Could you check a few things on this model? Use its own coordinates, in mm. A direction names the side the tool comes from. Round coordinates to 2 decimals unless told otherwise and drop trailing zeros. Write each loop counter-clockwise with the first axis right and the second up, starting at its lowest first coordinate (ties: lowest second). Pieces come first, ordered by that corner, then holes. Notation, with made-up numbers: (83.5, 50) -> (97.5, 50) arc R23 cw to (97.5, 61) -> close; hole circle Ø9 at (-34, -27). An arc over 180 degrees is marked (long way). One line per question, with ' | ' between items. Start each with the question number.
1. Imagine slicing it at B-B, the plane x = -85.5. List the corners of the cut face in (y, z) for me, and give its area (3 significant figures).
2. If I drill on line 1 along X through (y, z) = (0.75, -100); line 2 along X through (y, z) = (1.75, 70); line 3 along Z through (x, y) = (0, 1.8), over which ranges is the centre line in solid material (lowest first)? Write a range as [from, to].
3. For faces 1 (the flat face through (-95, 3, -95)), 2 (the flat face through (-53, 3, 123)), 3 (the flat face through (95, 3, -95)), 4 (the flat face through (85, 3, -105)), which set-ups out of +Z, -Z, +X, -X, +Y, -Y let a thin tool reach every point of the face, with its end or its side?
4. Thinking about a two-plate mould opening in X: for faces 5 (the flat face through (-90, 3, 120)), 6 (the flat face through (0, 3, -15)), 7 (the flat face through (-24, 0, -2)), which applies, released by +X, released by -X, zero draft, split by the parting line, or undercut?
5. Imagine slicing it at C-C, the plane y = 1.1. State how many separate pieces and enclosed holes the cut face has, and give its area (3 significant figures).
6. For pin 1 Ø2 at (x, y) = (-47, 1.5) entering from -Z; pin 2 Ø2.5 at (x, z) = (-20.61, 59.52) entering from -Y (1 decimal); pin 3 Ø2 at (x, y) = (-50, 4) entering from -Z, each with a flat end and sliding along its axis, tell me the tip position at first contact or that it passes through.
7. Imagine slicing it at A-A, the plane x = 5. List the corners of the cut face in (y, z) for me, and give its area (4 significant figures).
from build123d import *

# Parameters (mm, degrees)
SKETCH_1_W           = 200
SKETCH_1_H           = 250
EXTRUDE_1_DEPTH      = 5
CUT_EXTRUDE_1_DEPTH  = 35
CUT_EXTRUDE_2_DEPTH  = 35
CUT_EXTRUDE_3_DEPTH  = 35
CUT_EXTRUDE_5_DEPTH  = 30
CUT_EXTRUDE_6_DEPTH  = 10
CUT_EXTRUDE_7_DEPTH  = 10
SKETCH_9_R           = 1.5
CUT_EXTRUDE_8_DEPTH  = 10
SKETCH_10_R          = 1.5
CUT_EXTRUDE_9_DEPTH  = 10
SKETCH_12_R          = 1.5
CUT_EXTRUDE_10_DEPTH = 10
SKETCH_13_R          = 1.5
CUT_EXTRUDE_11_DEPTH = 10


with BuildPart() as part:
    # 草图1 → 凸台-拉伸1 (new body)
    with BuildSketch(Plane(origin=(0, 0, 0), x_dir=(1, 0, 0), z_dir=(0, 1, 0))):
        Rectangle(SKETCH_1_W, SKETCH_1_H)
    extrude(amount=EXTRUDE_1_DEPTH)

    # 草图2 → 切除-拉伸1 (cut)
    with BuildSketch(Plane(origin=(0, 5, 0), x_dir=(1, 0, 0), z_dir=(0, 1, 0))):
        Polygon((-100, -115), (-80, -125), (-100, -125), align=None)
    cut_extrude_1 = extrude(amount=-CUT_EXTRUDE_1_DEPTH, mode=Mode.SUBTRACT)

    # 镜向1: 切除-拉伸1 across plane
    add(cut_extrude_1.mirror(Plane(origin=(0, 0, 0), x_dir=(0, 0, 1), z_dir=(1, 0, 0))), mode=Mode.SUBTRACT)

    # 草图3 → 切除-拉伸2 (cut)
    with BuildSketch(Plane(origin=(0, 5, 0), x_dir=(1, 0, 0), z_dir=(0, 1, 0))):
        Polygon((-55, -125), (-50, -120), (0, -120), (0, -125), align=None)
    cut_extrude_2 = extrude(amount=-CUT_EXTRUDE_2_DEPTH, mode=Mode.SUBTRACT)

    # 镜向2: 切除-拉伸2 across plane
    add(cut_extrude_2.mirror(Plane(origin=(0, 0, 0), x_dir=(0, 0, 1), z_dir=(1, 0, 0))), mode=Mode.SUBTRACT)

    # 草图4 → 切除-拉伸3 (cut)
    with BuildSketch(Plane(origin=(0, 5, 0), x_dir=(1, 0, 0), z_dir=(0, 1, 0))):
        with BuildLine():
            Line((-12.5, -95), (12.5, -95))
            ThreePointArc((12.5, -95), (14.267766953, -95.732233047), (15, -97.5))
            Line((15, -97.5), (15, -107.5))
            ThreePointArc((15, -107.5), (14.267766953, -109.267766953), (12.5, -110))
            Line((12.5, -110), (-12.5, -110))
            ThreePointArc((-12.5, -110), (-14.267766953, -109.267766953), (-15, -107.5))
            Line((-15, -107.5), (-15, -97.5))
            ThreePointArc((-15, -97.5), (-14.267766953, -95.732233047), (-12.5, -95))
        make_face()
    extrude(amount=-CUT_EXTRUDE_3_DEPTH, mode=Mode.SUBTRACT)

    # 草图5 → 切除-拉伸5 (cut)
    with BuildSketch(Plane(origin=(0, 0, 0), x_dir=(1, 0, 0), z_dir=(0, 1, 0))):
        Polygon((-30, 125), (-100, 115), (-100, 125), align=None)
    cut_extrude_5 = extrude(amount=CUT_EXTRUDE_5_DEPTH, mode=Mode.SUBTRACT)

    # 镜向3: 切除-拉伸5 across plane
    add(cut_extrude_5.mirror(Plane(origin=(0, 0, 0), x_dir=(0, 0, 1), z_dir=(1, 0, 0))), mode=Mode.SUBTRACT)

    # 草图6 → 切除-拉伸6 (cut)
    with BuildSketch(Plane(origin=(0, 5, 0), x_dir=(1, 0, 0), z_dir=(0, 1, 0))):
        with BuildLine():
            Line((-100, 95), (-90, 95))
            Line((-90, 95), (-90, 105))
            Line((-90, 105), (-80, 105))
            ThreePointArc((-80, 105), (-75.121684822, 101.096376317), (-77.860612309, 95.480816412))
            Line((-77.860612309, 95.480816412), (-100, 85))
            Line((-100, 85), (-100, 95))
        make_face()
    cut_extrude_6 = extrude(amount=-CUT_EXTRUDE_6_DEPTH, mode=Mode.SUBTRACT)

    # 镜向4: 切除-拉伸6 across plane
    add(cut_extrude_6.mirror(Plane(origin=(0, 0, 0), x_dir=(0, 0, 1), z_dir=(1, 0, 0))), mode=Mode.SUBTRACT)

    # 草图8 → 切除-拉伸7 (cut)
    with BuildSketch(Plane(origin=(0, 5, 0), x_dir=(1, 0, 0), z_dir=(0, 1, 0))):
        with BuildLine():
            Line((-37.5, -45), (-27.5, -45))
            ThreePointArc((-27.5, -45), (-25.732233047, -45.732233047), (-25, -47.5))
            Line((-25, -47.5), (-25, -72.5))
            ThreePointArc((-25, -72.5), (-25.732233047, -74.267766953), (-27.5, -75))
            Line((-27.5, -75), (-37.5, -75))
            ThreePointArc((-37.5, -75), (-39.267766953, -74.267766953), (-40, -72.5))
            Line((-40, -72.5), (-40, -47.5))
            ThreePointArc((-40, -47.5), (-39.267766953, -45.732233047), (-37.5, -45))
        make_face()
        with BuildLine():
            Line((25, -47.5), (25, -72.5))
            ThreePointArc((25, -72.5), (25.732233047, -74.267766953), (27.5, -75))
            Line((27.5, -75), (37.5, -75))
            ThreePointArc((37.5, -75), (39.267766953, -74.267766953), (40, -72.5))
            Line((40, -72.5), (40, -47.5))
            ThreePointArc((40, -47.5), (39.267766953, -45.732233047), (37.5, -45))
            Line((37.5, -45), (27.5, -45))
            ThreePointArc((27.5, -45), (25.732233047, -45.732233047), (25, -47.5))
        make_face()
        with BuildLine():
            Line((-12.5, 15), (12.5, 15))
            ThreePointArc((12.5, 15), (14.267766953, 14.267766953), (15, 12.5))
            Line((15, 12.5), (15, 2.5))
            ThreePointArc((15, 2.5), (14.267766953, 0.732233047), (12.5, 0))
            Line((12.5, 0), (-12.5, 0))
            ThreePointArc((-12.5, 0), (-14.267766953, 0.732233047), (-15, 2.5))
            Line((-15, 2.5), (-15, 12.5))
            ThreePointArc((-15, 12.5), (-14.267766953, 14.267766953), (-12.5, 15))
        make_face()
    extrude(amount=-CUT_EXTRUDE_7_DEPTH, mode=Mode.SUBTRACT)

    # 草图9 → 切除-拉伸8 (cut)
    with BuildSketch(Plane(origin=(0, 5, 0), x_dir=(1, 0, 0), z_dir=(0, 1, 0))):
        with Locations((-80, -100)):
            Circle(SKETCH_9_R)
        with Locations((80, -100)):
            Circle(SKETCH_9_R)
    extrude(amount=-CUT_EXTRUDE_8_DEPTH, mode=Mode.SUBTRACT)

    # 草图10 → 切除-拉伸9 (cut)
    with BuildSketch(Plane(origin=(0, 5, 0), x_dir=(1, 0, 0), z_dir=(0, 1, 0))):
        with Locations((-80, 112.806380134)):
            Circle(SKETCH_10_R)
        with Locations((80, 112.806380134)):
            Circle(SKETCH_10_R)
    extrude(amount=-CUT_EXTRUDE_9_DEPTH, mode=Mode.SUBTRACT)

    # 草图12 → 切除-拉伸10 (cut)
    with BuildSketch(Plane(origin=(0, 5, 0), x_dir=(1, 0, 0), z_dir=(0, 1, 0))):
        with Locations((0, -38.912086487)):
            Circle(SKETCH_12_R)
        with Locations((-20.60616084, -59.518247327)):
            Circle(SKETCH_12_R)
        with Locations((20.60616084, -59.518247327)):
            Circle(SKETCH_12_R)
        with Locations((0, -80.124408167)):
            Circle(SKETCH_12_R)
    extrude(amount=-CUT_EXTRUDE_10_DEPTH, mode=Mode.SUBTRACT)

    # 草图13 → 切除-拉伸11 (cut)
    with BuildSketch(Plane(origin=(0, 5, 0), x_dir=(1, 0, 0), z_dir=(0, 1, 0))):
        with Locations((-50, -80)):
            Circle(SKETCH_13_R)
        with Locations((50, -80)):
            Circle(SKETCH_13_R)
        with Locations((-50, 50)):
            Circle(SKETCH_13_R)
        with Locations((50, 50)):
            Circle(SKETCH_13_R)
    extrude(amount=-CUT_EXTRUDE_11_DEPTH, mode=Mode.SUBTRACT)


solid = part.part
Geometry results:
1) outline: (0, -117.07) -> (5, -117.07) -> (5, -105) -> (0, -105) -> close; (0, -91.86) -> (5, -91.86) -> (5, 122.25) -> (0, 122.25) -> close | area: 1,130 mm2
2) line 1: x = [-100, -90], [-75, 75], [90, 100] | line 2: x = [-100, -40], [-25, 25], [40, 100] | line 3: z = [-125, -15], [0, 37.41], [40.41, 78.62], [81.62, 95], [110, 120]
3) face 1: -X, +Y, -Y | face 2: +Z, +Y, -Y | face 3: +X, +Y, -Y | face 4: +Y, -Y
4) face 5: released by -X | face 6: undercut | face 7: zero draft
5) separate pieces: 1 | enclosed holes: 16 | area: 46,200 mm2
6) pin 1: stops at z = -122.71 | pin 2: passes through | pin 3: stops at z = -122.29
7) outline: (0, -125) -> (5, -125) -> (5, -15) -> (0, -15) -> close; (0, 0) -> (5, 0) -> (5, 95) -> (0, 95) -> close; (0, 110) -> (5, 110) -> (5, 120) -> (0, 120) -> close | area: 1,075 mm2
